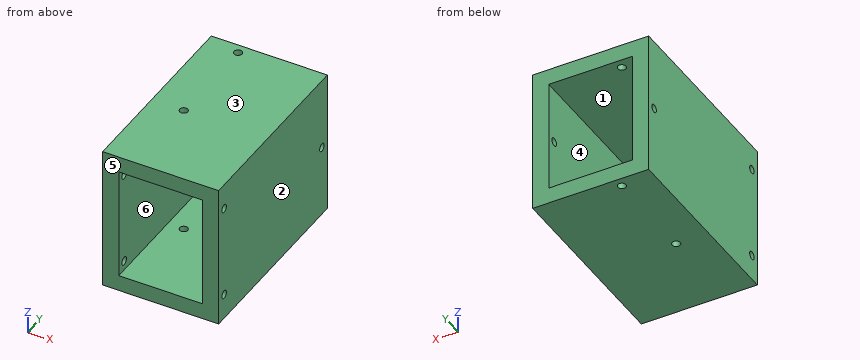
from build123d import *

# Parameters (mm, degrees)
SKETCH_1_W          = 36
SKETCH_1_H          = 45
SKETCH_1_W_2        = 26
SKETCH_1_H_2        = 35
EXTRUDE_1_DEPTH     = 60
SKETCH_4_R          = 1.25
CUT_EXTRUDE_1_DEPTH = 74.5
SKETCH_5_R          = 1.25
CUT_EXTRUDE_2_DEPTH = 78.129760793
SKETCH_6_R          = 1.25
CUT_EXTRUDE_3_DEPTH = 74.5


with BuildPart() as part:
    # 草图1 → 凸台-拉伸1 (new body)
    with BuildSketch(Plane(origin=(0, 0, 0), x_dir=(1, 0, 0), z_dir=(0, 1, 0))):
        Rectangle(SKETCH_1_W, SKETCH_1_H)
        Rectangle(SKETCH_1_W_2, SKETCH_1_H_2, mode=Mode.SUBTRACT)
    extrude(amount=EXTRUDE_1_DEPTH)

    # 草图4 → 切除-拉伸1 (cut, through all)
    with BuildSketch(Plane.ZY.offset(18)):
        with Locations((14.5, 3)):
            Circle(SKETCH_4_R)
        with Locations((-14.5, 3)):
            Circle(SKETCH_4_R)
    extrude(amount=-CUT_EXTRUDE_1_DEPTH, mode=Mode.SUBTRACT)

    # 草图5 → 切除-拉伸2 (cut, through all)
    with BuildSketch(Plane.XY.offset(22.5)):
        with Locations((-8, 57)):
            Circle(SKETCH_5_R)
        with Locations((-8, 27)):
            Circle(SKETCH_5_R)
    extrude(amount=-CUT_EXTRUDE_2_DEPTH, mode=Mode.SUBTRACT)

    # 草图6 → 切除-拉伸3 (cut, through all)
    with BuildSketch(Plane(origin=(18, 0, 0), x_dir=(0, 0, -1), z_dir=(1, 0, 0))):
        with Locations((0, 57)):
            Circle(SKETCH_6_R)
    extrude(amount=-CUT_EXTRUDE_3_DEPTH, mode=Mode.SUBTRACT)


solid = part.part
Source: CAD feature listing. Evaluate the final solid. Frame: model axes, mm. Face numbers are marked on the shaded views. A direction names the side the tool comes from. Coordinates: 2 decimals unless noted, no trailing zeros. Loops run counter-clockwise (first coordinate to the right, second up) from the corner with the lowest first, then second, coordinate; pieces in that order, holes last. Notation, with made-up numbers: M 72.5,31 L 127.5,31 A14 cw 127.5,54 Z; hole C 45,-6.5 d5. An arc over 180 degrees is marked long. Answer in a Markdown table with one row per item.
Q1. Draft query along Z for the marked faces 1, 2, 3 and 4. Return one class per face: pulls with the +Z half, pulls with the -Z half, needs draft (parallel to the pull), parting line crosses it, or undercut.
Answers below:
| item | result |
|---|---|
| face 1 | undercut |
| face 2 | needs draft |
| face 3 | pulls with the +Z half |
| face 4 | undercut |
Q2. Section D-D on x = 0.5. Return the cut outline in (y, z).
Answers below:
| item | result |
|---|---|
| outline | M 0,-22.5 L 60,-22.5 L 60,-17.5 L 0,-17.5 Z; M 0,17.5 L 60,17.5 L 60,22.5 L 0,22.5 Z |
Q3. First-contact query: pin 1 (10 mm diameter, centred on x = 5, z = 1.5, fed in from +Y); pin 2 (3 mm diameter, centred on y = 3, z = 14.5, fed in from -X). Flat tips, straight axial feed; report the tip coordinate or a pass-through.
Answers below:
| item | result |
|---|---|
| pin 1 | passes through |
| pin 2 | stops at x = -18 |
Q4. Ray query, probe 1 along Y at (x, z) = (-8, -20); probe 2 along Z at (x, y) = (9.5, 31); probe 3 along X at (y, z) = (46, -9.5). Return the intervals inside material, ascending. Write a range as from..to.
Answers below:
| item | result |
|---|---|
| probe 1 | y = 0..25.75, 28.25..55.75, 58.25..60 |
| probe 2 | z = -22.5..-17.5, 17.5..22.5 |
| probe 3 | x = -18..-13, 13..18 |
Q5. Set-up query: the marked faces 5 and 6. Return all of +Z, -Z, +X, -X, +Y, -Y with unobstructed straight access to the full face (end or side cutting, diameter ignored); none if empty.
Answers below:
| item | result |
|---|---|
| face 5 | +Z, -Z, +X, -X, -Y |
| face 6 | +Y, -Y |
Q6. Section C-C on z = 3. Return the cut outline in (x, y), plus the area to 3 significant figures.
Answers below:
| item | result |
|---|---|
| outline | M -18,0 L -13,0 L -13,60 L -18,60 Z; M 13,0 L 18,0 L 18,60 L 13,60 Z |
| area | 600 mm^2 |
Q7. Section B-B on z = -14.5. Return the cut outline in (x, y), plus the area to 3 significant figures.
Answers below:
| item | result |
|---|---|
| outline | M -18,0 L -13,0 L -13,1.75 L -18,1.75 Z; M -18,4.25 L -13,4.25 L -13,60 L -18,60 Z; M 13,0 L 18,0 L 18,1.75 L 13,1.75 Z; M 13,4.25 L 18,4.25 L 18,60 L 13,60 Z |
| area | 575 mm^2 |
Q8. Section A-A on y = 27. Return the cut outline in (x, z), plus the area to 3 significant figures.
Answers below:
| item | result |
|---|---|
| outline | M -18,-22.5 L -9.25,-22.5 L -9.25,-17.5 L -13,-17.5 L -13,17.5 L -9.25,17.5 L -9.25,22.5 L -18,22.5 Z; M -6.75,-22.5 L 18,-22.5 L 18,22.5 L -6.75,22.5 L -6.75,17.5 L 13,17.5 L 13,-17.5 L -6.75,-17.5 Z |
| area | 685 mm^2 |
